Design review of the part built by this model. Coordinates are the model's own, in mm. Face numbers are marked on the shaded views. A direction names the side the tool comes from. Give positions to 0.01 mm unless a question says otherwise; leave off trailing zeros. Order: outer loops, then holes, each group sorted by start corner. A loop starts at its lowest first (then second) coordinate and runs counter-clockwise, first axis right, second up.
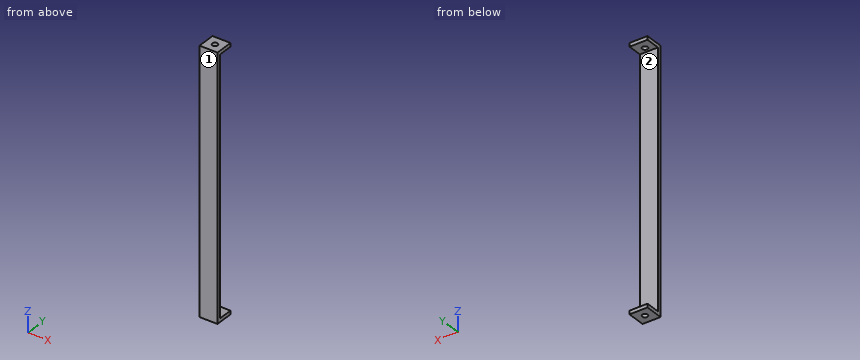
Autodesk Fusion 360 part; units mm, degrees
sketch "Sketch1" plane through (0, 0, 0) normal (0, 0, 1) x (1, 0, 0)
  line L0 (-14.9621, 7.481) -> (-4.9621, 7.481)
  line L1 (-4.9621, 7.481) -> (-4.9621, -2.519)
  line L2 (-4.9621, -2.519) -> (-14.9621, -2.519)
  line L3 (-14.9621, -2.519) -> (-14.9621, 7.481)
  line L4 (-14.9621, 7.481) -> (-9.9621, 7.481)
  line L5 (-14.9621, 7.481) -> (-9.9621, 7.481)
  line L6 (-9.9621, 7.481) -> (-9.9621, 2.481)
  line L7 (-4.9621, 7.481) -> (-9.9621, 7.481)
  circle A0 centre (-9.9621, 2.481) radius 1.5
  dimension "d1" = 10
  dimension "d2" = 10
  dimension "d3" = 5
  dimension "d4" = 3
extrude "Extrude1" add sketch "Sketch1" along normal blind 2
sketch "Sketch2" plane through (0, 0, 2) normal (0, 0, 1) x (1, 0, 0)
  circle A0 centre (-9.9621, 2.481) radius 1.5
  line L0 (-4.9621, -2.519) -> (-4.9621, 7.481)
  line L1 (-4.9621, 7.481) -> (-14.9621, 7.481)
  line L2 (-14.9621, 7.481) -> (-14.9621, -2.519)
  line L3 (-14.9621, -2.519) -> (-4.9621, -2.519)
  line L4 (-14.9621, -2.519) -> (-4.9621, -2.519)
  line L5 (-4.9621, -2.519) -> (-4.9621, -0.519)
  line L6 (-4.9621, -0.519) -> (-14.9621, -0.519)
  line L7 (-14.9621, -0.519) -> (-14.9621, -2.519)
  dimension "d7" = 10
  dimension "d8" = 2
extrude "Extrude2" add sketch "Sketch2" along normal blind 5 contours L0 L2 L3 L4 L5 L6 L7
extrude "Extrude3" add 1 faces at (-11.6287, -1.8523, 7) along direction (0, 0, 1) blind 136
sketch "Sketch3" plane through (0, 0, 143) normal (0, 0, 1) x (1, 0, 0)
  line L0 (-14.9621, -0.519) -> (-14.9621, -2.519)
  line L1 (-14.9621, -2.519) -> (-4.9621, -2.519)
  line L2 (-4.9621, -2.519) -> (-4.9621, -0.519)
  line L3 (-4.9621, -0.519) -> (-14.9621, -0.519)
  line L4 (-14.9621, -2.519) -> (-4.9621, -2.519)
  line L5 (-4.9621, -2.519) -> (-4.9621, 7.481)
  line L6 (-4.9621, 7.481) -> (-14.9621, 7.481)
  line L7 (-14.9621, 7.481) -> (-14.9621, -2.519)
  line L8 (-14.9621, -2.519) -> (-9.9621, -2.519)
  line L9 (-9.9621, -2.519) -> (-9.9621, 2.481)
  circle A0 centre (-9.9621, 2.481) radius 1.5
  dimension "d13" = 10
  dimension "d14" = 10
  dimension "d15" = 5
  dimension "d16" = 3
extrude "Extrude4" add sketch "Sketch3" along normal blind 2
1. Take a section at C-C (z = 52). State the section outline as (x, y) points, then the cut area to 3 significant figures.
Recorded:
outline: (-14.96, -2.52) - (-4.96, -2.52) - (-4.96, -0.52) - (-14.96, -0.52) - close
area: 20.0 mm2
2. Take a section at B-B (x = -6.25). State the section outline as (y, z) points, then the cut area to 3 significant figures.
Recorded:
outline: (-2.52, 0) - (7.48, 0) - (7.48, 2) - (-0.52, 2) - (-0.52, 143) - (7.48, 143) - (7.48, 145) - (-2.52, 145) - close
area: 322 mm2
3. Machinability: for the marked faces 1 and 2, which of the approach directions +Z, -Z, +X, -X, +Y, -Y give a long, thin tool a straight path to every point of the face, cutting with its end or side? Answer none if there is none.
Recorded:
face 1: +Z, -Z, +X, -X, -Y
face 2: +X, -X, +Y
4. For line 1 along Z through (x, y) = (-8.75, 3.5); line 2 along Y through (x, z) = (-6.25, 73), list the stretches that pass through material, from the lowest coordinate up.
Recorded:
line 1: z = 0 to 2, 143 to 145
line 2: y = -2.52 to -0.52
5. For pin 1 (1.8 mm diameter, centred on x = -9.96, y = 2.48, fed in from +Z); pin 2 (2 mm diameter, centred on x = -9.5, y = 6, fed in from -Z); pin 3 (5 mm diameter, centred on x = -11.5, z = 39.5, fed in from +Y), all flat-tipped, find the tip position at first contact; note any pin that passes through.
Recorded:
pin 1: passes through
pin 2: stops at z = 0
pin 3: stops at y = -0.52
6. Take a section at A-A (y = 5.75). State the section outline as (x, z) points.
Recorded:
outline: (-14.96, 0) - (-4.96, 0) - (-4.96, 2) - (-14.96, 2) - close; (-14.96, 143) - (-4.96, 143) - (-4.96, 145) - (-14.96, 145) - close
